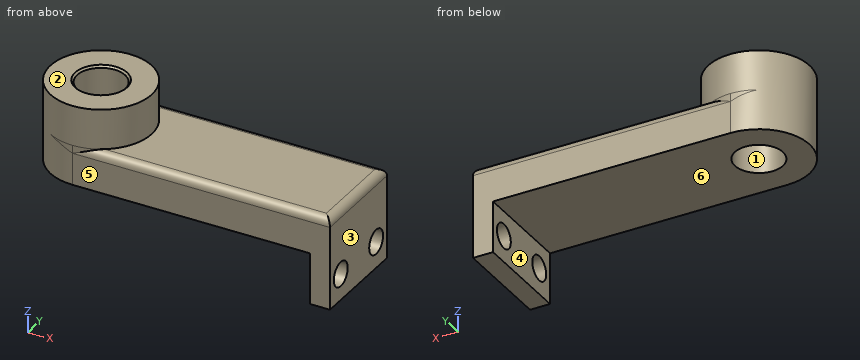
from build123d import *

# Parameters (mm, degrees)
F1_DEPTH     = 25.4
F2_DEPTH     = 50.8
F3_W         = 64.2605721951
F3_H         = 58.0011609286
F3_R         = 7.8158537252
F4_DEPTH     = 12.7
F5_T1_DEPTH  = 89.6605721951
F5_T6_DEPTH  = 197.5881144994
F5_S7_R      = 32.1302860975
F5_T8_DEPTH  = 100
F5_T12_DEPTH = 197.5881144994
F5_S13_R     = 32.1302860975
F5_T14_DEPTH = 100


# Not quite as in the source:
# - a fillet or chamfer that OpenCascade refuses, or shapes differently, is made with other operations: its cross-section is extruded or revolved along the edge and cut away or added


with BuildPart() as f1:
    # F0 (on Top) → F1 (new body)
    with BuildSketch(Plane.XY):
        with BuildLine():
            Line((81.6490572497, -32.1302860975), (81.6490572497, 32.1302860975))
            Line((81.6490572497, 32.1302860975), (-81.6490572497, 32.1302860975))
            ThreePointArc((-81.6490572497, 32.1302860975), (-58.9295140687, 22.719543181), (-49.5187711522, 0))
            ThreePointArc((-49.5187711522, 0), (-58.9295140687, -22.719543181), (-81.6490572497, -32.1302860975))
            Line((-81.6490572497, -32.1302860975), (81.6490572497, -32.1302860975))
        make_face()
        with BuildLine():
            Line((-81.6490572497, 15.24), (-81.6490572497, 32.1302860975))
            ThreePointArc((-81.6490572497, 32.1302860975), (-113.7793433473, 0), (-81.6490572497, -32.1302860975))
            Line((-81.6490572497, -32.1302860975), (-81.6490572497, -15.24))
            ThreePointArc((-81.6490572497, -15.24), (-96.8890572497, 0), (-81.6490572497, 15.24))
        make_face()
        with BuildLine():
            ThreePointArc((-49.5187711522, 0), (-58.9295140687, 22.719543181), (-81.6490572497, 32.1302860975))
            Line((-81.6490572497, 32.1302860975), (-81.6490572497, 15.24))
            ThreePointArc((-81.6490572497, 15.24), (-70.8727499044, 10.7763073453), (-66.4090572497, 0))
            ThreePointArc((-66.4090572497, 0), (-70.8727499044, -10.7763073453), (-81.6490572497, -15.24))
            Line((-81.6490572497, -15.24), (-81.6490572497, -32.1302860975))
            ThreePointArc((-81.6490572497, -32.1302860975), (-58.9295140687, -22.719543181), (-49.5187711522, 0))
        make_face()
    extrude(amount=F1_DEPTH)

    # F0 (on Top) → F2 (join)
    with BuildSketch(Plane.XY):
        with BuildLine():
            Line((-81.6490572497, 15.24), (-81.6490572497, 32.1302860975))
            ThreePointArc((-81.6490572497, 32.1302860975), (-113.7793433473, 0), (-81.6490572497, -32.1302860975))
            Line((-81.6490572497, -32.1302860975), (-81.6490572497, -15.24))
            ThreePointArc((-81.6490572497, -15.24), (-96.8890572497, 0), (-81.6490572497, 15.24))
        make_face()
        with BuildLine():
            ThreePointArc((-49.5187711522, 0), (-58.9295140687, 22.719543181), (-81.6490572497, 32.1302860975))
            Line((-81.6490572497, 32.1302860975), (-81.6490572497, 15.24))
            ThreePointArc((-81.6490572497, 15.24), (-70.8727499044, 10.7763073453), (-66.4090572497, 0))
            ThreePointArc((-66.4090572497, 0), (-70.8727499044, -10.7763073453), (-81.6490572497, -15.24))
            Line((-81.6490572497, -15.24), (-81.6490572497, -32.1302860975))
            ThreePointArc((-81.6490572497, -32.1302860975), (-58.9295140687, -22.719543181), (-49.5187711522, 0))
        make_face()
    extrude(amount=F2_DEPTH)

    # F3 (on face) → F4 (join)
    with BuildSketch(Plane.YZ.offset(81.6490572497)):
        with Locations((0, -3.6005804643)):
            Rectangle(F3_W, F3_H)
        with Locations((-19.9125986546, -15.9243624657)):
            Circle(F3_R, mode=Mode.SUBTRACT)
        with Locations((19.9125986546, -15.9243624657)):
            Circle(F3_R, mode=Mode.SUBTRACT)
    extrude(amount=-F4_DEPTH)

    # F5: fillet of radius 5.08 on 3 edges, made by hand

    # F5_s2 → F5_t1 (cut)
    with BuildSketch(Plane.XZ.offset(-44.8302860975)):
        with BuildLine():
            ThreePointArc((81.6490572497, 20.32), (80.1611596982, 23.9121024484), (76.5690572497, 25.4))
            Line((76.5690572497, 25.4), (81.6490572497, 25.4))
            Line((81.6490572497, 25.4), (81.6490572497, 20.32))
        make_face()
    extrude(amount=F5_T1_DEPTH, mode=Mode.SUBTRACT)


with BuildPart() as f5_tool4:
    # F5_s5 → F5_t6 (new body)
    with BuildSketch(Plane.YZ.offset(94.3490572497)):
        with BuildLine():
            ThreePointArc((-27.0502860975, 25.4), (-30.642388546, 23.9121024484), (-32.1302860975, 20.32))
            Line((-32.1302860975, 20.32), (-32.1302860975, 25.4))
            Line((-32.1302860975, 25.4), (-27.0502860975, 25.4))
        make_face()
    extrude(amount=-F5_T6_DEPTH)

    # F5_s7 → F5_t8 (cut, symmetric)
    with BuildSketch(Plane.XY.offset(22.9)):
        with Locations((-81.6490572497, 0)):
            Circle(F5_S7_R)
    extrude(amount=F5_T8_DEPTH, both=True, mode=Mode.SUBTRACT)


with BuildPart() as f1_1:
    add(f1.part)

    # F5_t3: cut F5_tool4
    add(f5_tool4.part, mode=Mode.SUBTRACT)


with BuildPart() as f5_tool10:
    # F5_s11 → F5_t12 (new body)
    with BuildSketch(Plane.YZ.offset(-103.2390572497)):
        with BuildLine():
            ThreePointArc((32.1302860975, 20.32), (30.642388546, 23.9121024484), (27.0502860975, 25.4))
            Line((27.0502860975, 25.4), (32.1302860975, 25.4))
            Line((32.1302860975, 25.4), (32.1302860975, 20.32))
        make_face()
    extrude(amount=F5_T12_DEPTH)

    # F5_s13 → F5_t14 (cut, symmetric)
    with BuildSketch(Plane.XY.offset(22.9)):
        with Locations((-81.6490572497, 0)):
            Circle(F5_S13_R)
    extrude(amount=F5_T14_DEPTH, both=True, mode=Mode.SUBTRACT)


with BuildPart() as f1_2:
    add(f1_1.part)

    # F5_t9: cut F5_tool10
    add(f5_tool10.part, mode=Mode.SUBTRACT)

    # F6: chamfer of 1.27 on 1 edges, made by hand

    # F6_s1 → F6_t2 (revolve, cut)
    with BuildSketch(Plane.YZ.offset(-81.6490572497)):
        Polygon((15.24, 49.53), (16.51, 50.8), (15.24, 50.8), align=None)
    revolve(axis=Axis((-81.6490572497, 0, 50.8), (0, 0, -1)), mode=Mode.SUBTRACT)


solid = f1_2.part
The listing builds one solid part. Answer for the finished solid, in the listing's coordinates (mm). Face numbers are marked on the shaded views. A direction names the side the tool comes from. Give positions to 0.01 mm unless a question says otherwise; leave off trailing zeros. Loops run counter-clockwise (first coordinate to the right, second up) from the corner with the lowest first, then second, coordinate; pieces in that order, holes last. Notation, with made-up numbers: (7, 34.5) - (39, 34.5) arc R38 ccw to (39, 72.5) - close; hole circle Ø10 at (10.5, -39.75). An arc over 180 degrees is marked (long way). Use one line per item in the form item = value.
1. Section C-C on x = 11 is taken. Give the vertices of the cut face in (y, z), then the cut area to 3 significant figures.
Calculated:
outline = (-32.13, 0) - (32.13, 0) - (32.13, 20.32) arc R5.08 ccw to (27.05, 25.4) - (-27.05, 25.4) arc R5.08 ccw to (-32.13, 20.32) - close
area = 1,620 mm^2
2. Given pin 1 Ø2 at (x, y) = (-39.5, 18.5) entering from -Z; pin 2 Ø10 at (y, z) = (-8, -15) entering from -X; pin 3 Ø5 at (y, z) = (-15, -15.5) entering from +X; pin 4 Ø6 at (x, y) = (33, -2.5) entering from +Z, each flat-ended and moving along its own axis, determine where each tip first touches the part or whether it passes through.
Calculated:
pin_1 = 0
pin_2 = 68.95
pin_3 = through
pin_4 = 25.4
3. Section B-B on z = -21.5 is taken. Give the vertices of the cut face in (x, y), then the cut area to 3 significant figures.
Calculated:
outline = (68.95, -32.13) - (81.65, -32.13) - (81.65, -25.39) - (68.95, -25.39) - close; (68.95, -14.44) - (81.65, -14.44) - (81.65, 14.44) - (68.95, 14.44) - close; (68.95, 25.39) - (81.65, 25.39) - (81.65, 32.13) - (68.95, 32.13) - close
area = 538 mm^2
4. Which of the six approach directions +Z, -Z, +X, -X, +Y, -Y give full straight-line access (tool end or side, diameter ignored) to the marked faces 5 and 6?
Calculated:
face_5 = +Z, -Z, +X, -X, -Y
face_6 = -Z, -X, +Y, -Y
5. Find the intervals of material crossed by line 1 along X through (y, z) = (0, 31); line 2 along Z through (x, y) = (-18.5, -13); line 3 along Z through (x, y) = (-103.5, 10), in increasing order. Write a range as [from, to].
Calculated:
line_1 = [-113.78, -96.89], [-66.41, -49.52]
line_2 = [0, 25.4]
line_3 = [0, 50.8]
6. Section D-D on x = -55 is taken. Give the vertices of the cut face in (y, z), then the cut area to 3 significant figures.
Calculated:
outline = (-32.13, 0) - (32.13, 0) - (32.13, 20.32) arc R5.08 ccw to (27.05, 25.4) - (17.95, 25.4) - (17.95, 50.8) - (-17.95, 50.8) - (-17.95, 25.4) - (-27.05, 25.4) arc R5.08 ccw to (-32.13, 20.32) - close
area = 2,530 mm^2
7. Section A-A on y = 0 is taken. Give the vertices of the cut face in (x, z), then the cut area to 3 significant figures.
Calculated:
outline = (-113.78, 0) - (-96.89, 0) - (-96.89, 49.53) - (-98.16, 50.8) - (-113.78, 50.8) - close; (-66.41, 0) - (68.95, 0) - (68.95, -32.6) - (81.65, -32.6) - (81.65, 20.32) arc R5.08 ccw to (76.57, 25.4) - (-49.52, 25.4) - (-49.52, 50.8) - (-65.14, 50.8) - (-66.41, 49.53) - close
area = 5,450 mm^2
8. The mould has two halves that part along X. Classify the marked faces 1, 2, 3 and 4: pulls with the +X half, pulls with the -X half, needs draft (parallel to the pull), parting line crosses it, or undercut.
Calculated:
face_1 = undercut
face_2 = needs draft
face_3 = pulls with the +X half
face_4 = pulls with the -X half
